The model under review builds one solid part; all positions refer to its coordinate system, in mm. A direction names the side the tool comes from. Round coordinates to 2 decimals unless told otherwise and drop trailing zeros. Write each loop counter-clockwise with the first axis right and the second up, starting at its lowest first coordinate (ties: lowest second). Pieces come first, ordered by that corner, then holes. Notation, with made-up numbers: (32, 0) -> (71, 0) arc R23 ccw to (71, 18) -> close; hole circle Ø5 at (76, 31.25). An arc over 180 degrees is marked (long way). Use CSV: the item, a comma, the result in double quotes. Start each with the question number.
1) Take a section at A-A, the plane z = 44.9. Give the boundary of the cut face in (x, y), then the cut area to 3 significant figures.
2) Machinability: for faces 4 (the face through (-30.852, -35, 43)), 5 (the face through (-30.599, -64.923, 43.186)), which of the approach directions +Z, -Z, +X, -X, +Y, -Y give a long, thin tool a straight path to every point of the face, cutting with its end or side? Answer none if there is none.
3) Take a section at C-C, the plane y = -41. Give the boundary of the cut face in (x, z).
4) Take a section at B-B, the plane y = -57.5. Give the boundary of the cut face in (x, z).
5) Wall thickness on probe 1 along X at (y, z) = (-29.5, 45.2); probe 2 along Z at (x, y) = (-52, -33); probe 3 along Y at (x, z) = (-38.5, 46): over which ranges is each line inside the solid? List them lowest first. Write a range as [from, to].
6) Take a section at D-D, the plane x = -52. Give the boundary of the cut face in (y, z), then the cut area to 3 significant figures.
7) For pin 1 Ø0.6 at (x, y) = (-61, -8) entering from +Z; pin 2 Ø2 at (x, y) = (-38, -45) entering from -Z; pin 3 Ø10 at (x, y) = (-35.5, -33.5) entering from -Z; pin 4 Ø0.6 at (x, z) = (-51, 46) entering from -Y, all flat-tipped, find the tip position at first contact; note any pin that passes through.
8) Mouldability with a two-part tool opening along X and no side actions: class faces 1 (the face through (-30.599, -6.285, 42.191)), 2 (the face through (-61.352, -35, 44)), 3 (the face through (-46, -35, 45.753)) as released by +X, released by -X, zero draft, split by the parting line, or undercut.
from build123d import *

# Parameters (mm, degrees)
F0_W     = 0.5
F0_H     = 5
F1_DEPTH = 70
F2_DEPTH = 25
F3_START = 45
F3_DEPTH = 25
F4_R     = 1
F5_DEPTH = 84.25
F6_R     = 1
F7_DEPTH = 160.25


with BuildPart() as f1:
    # F0 (on Front) → F1 (new body)
    with BuildSketch(Plane.XZ):
        with Locations((-61.1022742987, 43.2528425008)):
            Rectangle(F0_W, F0_H)
        Polygon((-61.3522742987, 45.7528425008), (-60.8522742987, 45.7528425008), (-30.8522742987, 45.7528425008), (-30.3522742987, 45.7528425008), (-30.3522742987, 46.2528425008), (-61.3522742987, 46.2528425008), align=None)
        with Locations((-30.6022742987, 43.2528425008)):
            Rectangle(F0_W, F0_H)
    extrude(amount=F1_DEPTH)

    # F0 (on Front) → F2 (cut)
    with BuildSketch(Plane.XZ):
        Polygon((-61.3522742987, 45.7528425008), (-60.8522742987, 45.7528425008), (-30.8522742987, 45.7528425008), (-30.3522742987, 45.7528425008), (-30.3522742987, 46.2528425008), (-61.3522742987, 46.2528425008), align=None)
    extrude(amount=F2_DEPTH, mode=Mode.SUBTRACT)

    # F0 (on Front) → F3 (cut)
    with BuildSketch(Plane.XZ.offset(F3_START)):
        Polygon((-61.3522742987, 45.7528425008), (-60.8522742987, 45.7528425008), (-30.8522742987, 45.7528425008), (-30.3522742987, 45.7528425008), (-30.3522742987, 46.2528425008), (-61.3522742987, 46.2528425008), align=None)
    extrude(amount=F3_DEPTH, mode=Mode.SUBTRACT)

    # F4 (on Right) → F5 (cut)
    with BuildSketch(Plane.YZ):
        with Locations((-63.924215734, 43.1419759989)):
            Circle(F4_R)
    extrude(amount=-F5_DEPTH, mode=Mode.SUBTRACT)

    # F6 (on Right) → F7 (cut)
    with BuildSketch(Plane.YZ):
        with Locations((-6.0686194338, 43.1675091386)):
            Circle(F6_R)
    extrude(amount=-F7_DEPTH, mode=Mode.SUBTRACT)


solid = f1.part
Values found:
1,outline,"(-61.35, -70) -> (-60.85, -70) -> (-60.85, 0) -> (-61.35, 0) -> close; (-30.85, -70) -> (-30.35, -70) -> (-30.35, 0) -> (-30.85, 0) -> close"
1,area,"70.0 mm²"
2,face 4,"-Z, +Y, -Y"
2,face 5,"+X, -X"
3,outline,"(-61.35, 40.75) -> (-60.85, 40.75) -> (-60.85, 45.75) -> (-30.85, 45.75) -> (-30.85, 40.75) -> (-30.35, 40.75) -> (-30.35, 46.25) -> (-61.35, 46.25) -> close"
4,outline,"(-61.35, 40.75) -> (-60.85, 40.75) -> (-60.85, 45.75) -> (-61.35, 45.75) -> close; (-30.85, 40.75) -> (-30.35, 40.75) -> (-30.35, 45.75) -> (-30.85, 45.75) -> close"
5,probe 1,"[-61.35, -60.85], [-30.85, -30.35]"
5,probe 2,"[45.75, 46.25]"
5,probe 3,"[-45, -25]"
6,outline,"(-45, 45.75) -> (-25, 45.75) -> (-25, 46.25) -> (-45, 46.25) -> close"
6,area,"10.0 mm²"
7,pin 1,"z = 45.75"
7,pin 2,"z = 45.75"
7,pin 3,"z = 40.75"
7,pin 4,"y = -45"
8,face 1,"zero draft"
8,face 2,"released by -X"
8,face 3,"undercut"
